Autodesk Inventor part; units mm, degrees
ref_plane "YZ Plane" through (0, 0, 0) normal (1, 0, 0) x (0, 1, 0)
ref_plane "XZ Plane" through (0, 0, 0) normal (0, 1, 0) x (-1, 0, 0)
ref_plane "XY Plane" through (0, 0, 0) normal (0, 0, 1) x (1, 0, 0)
sketch "Sketch1" plane through (0, 0, 0) normal (0, 1, 0) x (-1, 0, 0)
  line L0 (-1.5, 6) -> (1.5, 6)
  line L1 (1.5, 6) -> (1.5, -6)
  line L2 (1.5, -6) -> (-1.5, -6)
  line L3 (-1.5, -6) -> (-1.5, 6)
  line L4 (-1.5, 6) -> (1.5, -6) construction
  line L5 (1.5, 6) -> (-1.5, -6) construction
  point P0 (0, 0)
  dimension "d0" = 3
  dimension "d1" = 12
extrude "Extrusion1" add sketch "Sketch1" along normal blind 28.5
fillet "Fillet1" radius 6 2 edges at (0, 28.5, 6) (0, 28.5, -6)
sketch "Sketch4" plane through (1.5, 0, 6) normal (1, 0, 0) x (0, 0, -1)
  arc A0 (12, 22.5) -> (0, 22.5) centre (6, 22.5) ccw
  circle A1 centre (6, 22.5) radius 4
  point P0 (6, 0)
  dimension "d14" = 8
extrude "Extrusion4" cut sketch "Sketch4" against normal through all
properties part number "middleLegv2-1_3DPrint"
Geometry: final body of the model. Coordinates: model frame, mm. Coordinates: 2 decimals unless noted, no trailing zeros. Loops run counter-clockwise (first coordinate to the right, second up) from the corner with the lowest first, then second, coordinate; pieces in that order, holes last. Notation, with made-up numbers: (-37, 47) - (22, 47) arc R33 ccw to (22, 76) - close; hole circle Ø6 at (43, 54.25). An arc over 180 degrees is marked (long way). One line per question, with ' | ' between items. Start each with the question number.
(1) Draft query along Z for faces 1 (the flat face through (0, 0, 0)), 2 (the cylindrical face through (-0.021, 26.696, 4.289)), 3 (the cylindrical face through (0.021, 26.466, 0.521)). Return one class per face: +Z half, -Z half, draft (parallel to the pull), parting line (faces both ways), or undercut.
(2) Cut plane B-B on z = 3.25. Output: boundary loops of the cut face in (x, y), and give its area (3 significant figures).
(3) Ray query, L1, parallel to Y at x = -0.1, z = 0; L2, parallel to Y at x = -1.15, z = 1.5; L3, parallel to Z at x = 0.65, y = 25.5. Return the intervals inside material, ascending. Write a range as from..to.
(4) Cut plane C-C on z = 4.5. Output: boundary loops of the cut face in (x, y).
Here are the results:
1) face 1: draft | face 2: +Z half | face 3: undercut
2) outline: (-1.5, 0) - (1.5, 0) - (1.5, 20.17) - (-1.5, 20.17) - close; (-1.5, 24.83) - (1.5, 24.83) - (1.5, 27.54) - (-1.5, 27.54) - close | area: 68.6 mm²
3) L1: 0..18.5, 26.5..28.5 | L2: 0..18.79, 26.21..28.31 | L3: -5.2..-2.65, 2.65..5.2
4) outline: (-1.5, 0) - (1.5, 0) - (1.5, 26.47) - (-1.5, 26.47) - close
